Can you work these out from the model? Positions are in its coordinate system, mm. A direction names the side the tool comes from. Round coordinates to 2 decimals unless told otherwise and drop trailing zeros. Order: outer loops, then holes, each group sorted by start corner. A loop starts at its lowest first (then second) coordinate and runs counter-clockwise, first axis right, second up.
Q1. If we section it at D-D (y = 3.75): Please give me the cut outline in (x, z).
Q2. If we section it at B-B (x = 0): Please give me the cut outline in (y, z), plus the area to 3 significant figures.
Q3. If I drill on line 1 (X direction, y = 1.05, z = 0); line 2 (X direction, y = 7.5, z = -5.5); line 3 (Z direction, x = 0, y = 1.1), over which ranges is the centre line in solid material (lowest first)?
Q4. If we section it at A-A (z = 8.75): Please give me the cut outline in (x, y).
Q5. We'd pull the mould along X, two halves only. Please class faces 1 (the face through (0, 15, 0)), 2 (the face through (1.425, 10.07, 8.174)), 3 (the face through (-10.6, 9.9, 0)), 4 (the face through (10.6, 9.9, 0)): pulls with the +X half, pulls with the -X half, needs draft (parallel to the pull), parting line crosses it, or undercut.
Q6. For faces 5 (the face through (3, 5, -5)), 6 (the face through (8.6, 9.9, 6.2)), 7 (the face through (5.589, 2.465, 2.317)), which set-ups out of +Z, -Z, +X, -X, +Y, -Y let a thin tool reach every point of the face, with its end or its side?
Q7. If we section it at C-C (z = 0): Please give me the cut outline in (x, y), plus the area to 3 significant figures.
Q8. Will these pins go through, and if not, where does the flat tip stop? P1, Ø1, axis at x = 8.5, z = -2, coming from the +Y side; P2, Ø1.5, axis at x = -3.5, y = 9, coming from the +Z side; P3, Ø1.2, axis at x = 6.5, z = 4.5, coming from the -Y side; P4, Ø0.7, axis at x = 3.5, z = -5, coming from the +Y side.
from build123d import *

# Parameters (mm, degrees)
SKETCH1_R           = 6.05
BOSS_EXTRUDE1_DEPTH = 5
SKETCH2_R           = 10.6
BOSS_EXTRUDE2_DEPTH = 10
CUT_EXTRUDE1_DEPTH  = 10
CIRPATTERN1_COUNT   = 10


with BuildPart() as part:
    # Sketch1 → Boss-Extrude1 (new body)
    with BuildSketch(Plane(origin=(0, 0, 0), x_dir=(1, 0, 0), z_dir=(0, 1, 0))):
        Circle(SKETCH1_R)
        with BuildLine():
            Line((-1.6, 2.596632435), (1.6, 2.596632435))
            ThreePointArc((1.6, 2.596632435), (0, -3.05), (-1.6, 2.596632435))
        make_face(mode=Mode.SUBTRACT)
    extrude(amount=BOSS_EXTRUDE1_DEPTH)

    # Sketch2 → Boss-Extrude2 (add)
    with BuildSketch(Plane(origin=(0, 5, 0), x_dir=(1, 0, 0), z_dir=(0, 1, 0))):
        Circle(SKETCH2_R)
    extrude(amount=BOSS_EXTRUDE2_DEPTH)

    # Sketch3 → Cut-Extrude1 (cut)
    with BuildSketch(Plane(origin=(0, 15, 0), x_dir=(1, 0, 0), z_dir=(0, 1, 0))):
        with BuildLine():
            Line((0.705423459, 5.6), (-0.705423459, 5.6))
            ThreePointArc((-0.705423459, 5.6), (-0.913686499, 5.684068284), (-1.00522743, 5.889156627))
            ThreePointArc((-1.00522743, 5.889156627), (-3.446318924, 11.358179096), (-9, 13.6))
            Line((-9, 13.6), (9, 13.6))
            ThreePointArc((9, 13.6), (3.446318924, 11.358179096), (1.00522743, 5.889156627))
            ThreePointArc((1.00522743, 5.889156627), (0.913686499, 5.684068284), (0.705423459, 5.6))
        make_face()
    cut_extrude1 = extrude(amount=-CUT_EXTRUDE1_DEPTH, mode=Mode.SUBTRACT)

    # CirPattern1: Cut-Extrude1 ×10 about axis
    cirpattern1_axis = Axis((0, 0, 0), (0, 1, 0))
    for i in range(1, CIRPATTERN1_COUNT):
        add(cut_extrude1.rotate(cirpattern1_axis, i * 360 / CIRPATTERN1_COUNT), mode=Mode.SUBTRACT)


solid = part.part
Solution:
1. outline: circle Ø12.1 at (0, 0); hole (-1.6, -2.6) - (1.6, -2.6) arc R3.05 ccw (long way) to start
2. outline: (0, -6.05) - (5, -6.05) - (5, -5.6) - (15, -5.6) - (15, 5.6) - (5, 5.6) - (5, 6.05) - (0, 6.05) - (0, 3.05) - (5, 3.05) - (5, -2.6) - (0, -2.6) - close
2. area: 144 mm2
3. line 1: x = -6.05 to -3.05, 3.05 to 6.05
3. line 2: x = -8.95 to -5.59, -2.74 to 2.74, 5.59 to 8.95
3. line 3: z = -6.05 to -2.6, 3.05 to 6.05
4. outline: (-3.94, 5) - (-1.65, 5) - (-1.65, 15) - (-3.94, 15) - close; (1.65, 5) - (3.94, 5) - (3.94, 15) - (1.65, 15) - close
5. face 1: needs draft
5. face 2: undercut
5. face 3: pulls with the -X half
5. face 4: pulls with the +X half
6. face 5: +Y
6. face 6: +Z, +X, +Y, -Y
6. face 7: -Y
7. outline: (-10.6, 5) - (-6.05, 5) - (-6.05, 0) - (-3.05, 0) - (-3.05, 5) - (3.05, 5) - (3.05, 0) - (6.05, 0) - (6.05, 5) - (10.6, 5) - (10.6, 15) - (-10.6, 15) - close
7. area: 242 mm2
8. P1: passes through
8. P2: stops at z = 10.24
8. P3: stops at y = 5
8. P4: stops at y = 5
